Here's how the part is built. I have some questions about the finished solid (model axes, mm). Round coordinates to 2 decimals unless told otherwise and drop trailing zeros. One line per item, written item: value. Start each with the question number.
```python
from build123d import *

# Parameters (mm, degrees)
SKETCH1_R           = 25
SKETCH1_R_2         = 3.75
SKETCH1_W           = 3.2
SKETCH1_H           = 1.7
BOSS_EXTRUDE1_DEPTH = 1
FILLET1_R           = 2
FILLET2_R           = 1


with BuildPart() as part:
    # Sketch1 → Boss-Extrude1 (new body)
    with BuildSketch(Plane(origin=(0, 0, 0), x_dir=(1, 0, 0), z_dir=(0, 1, 0))):
        with Locations(Location((0, 0, 0), (0, 0, 270))):
            Circle(SKETCH1_R)
        with Locations(Location((0, 0, 0), (0, 0, 270))):
            Circle(SKETCH1_R_2, mode=Mode.SUBTRACT)
        with BuildLine():
            Line((-5, -11.456439237), (-5, -16.770509831))
            ThreePointArc((-5, -16.770509831), (0, 17.5), (5, -16.770509831))
            Line((5, -16.770509831), (5, -11.456439237))
            ThreePointArc((5, -11.456439237), (0, 12.5), (-5, -11.456439237))
        make_face(mode=Mode.SUBTRACT)
        with Locations((0, -7.85)):
            Rectangle(SKETCH1_W, SKETCH1_H, mode=Mode.SUBTRACT)
    extrude(amount=BOSS_EXTRUDE1_DEPTH)

    # Fillet1
    fillet1_edges = [part.edges().sort_by_distance(p)[0] for p in [
        (-5, 0.5, 11.456439237),
        (5, 0.5, 11.456439237),
        (5, 0.5, 16.770509831),
        (-5, 0.5, 16.770509831),
    ]]
    fillet(fillet1_edges, radius=FILLET1_R)

    # Fillet2
    fillet2_edges = [part.edges().sort_by_distance(p)[0] for p in [
        (5.952730124, 0, 15.533202189),
        (5, 0, 13.263870893),
        (5.277932277, 0, 11.681329844),
        (0, 0, -12.5),
        (-5.277932277, 0, 11.681329844),
        (-5, 0, 13.263870893),
        (-5.952730124, 0, 15.533202189),
        (0, 0, -17.5),
        (0, 0, -25),
    ]]
    fillet(fillet2_edges, radius=FILLET2_R - 0.0001)  # a hair under: the kernel refuses the full size


solid = part.part
```
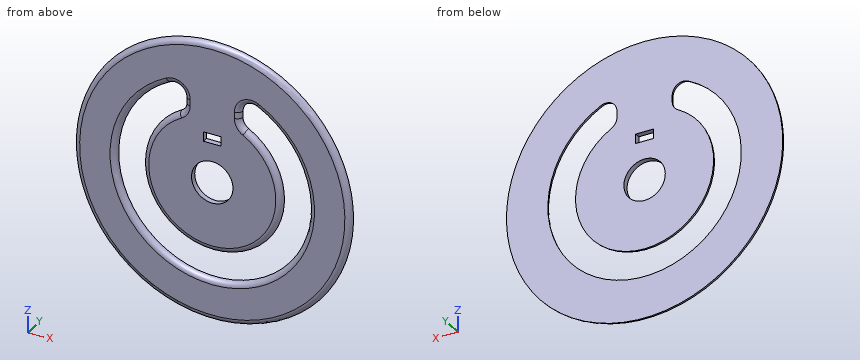
Q1. Will these pins go through, and if not, where does the flat tip stop? P1, Ø12, axis at x = 14, z = -6, coming from the +Y side; P2, Ø0.5, axis at y = 0.5, z = 8, coming from the -X side.
Q2. I want a section at A-A on x = 0. State how many separate pieces and enclosed holes the cut face has, plus the area to 3 significant figures.
Q3. If I drill on line 1 along X through (y, z) = (0.85, 0); line 2 along Z through (x, y) = (1, 0.55); line 3 along X through (y, z) = (0.45, 0), over which ranges is the centre line in solid material (lowest first)?
Answers below:
1. P1: stops at y = 1
1. P2: stops at x = -23.69
2. separate pieces: 4
2. enclosed holes: 0
2. area: 34.9 mm^2
3. line 1: x = -24.99 to -17.51, -12.49 to -3.75, 3.75 to 12.49, 17.51 to 24.99
3. line 2: z = -24.87 to -17.58, -12.35 to -3.61, 3.61 to 7, 8.7 to 24.87
3. line 3: x = -24.84 to -17.66, -12.34 to -3.75, 3.75 to 12.34, 17.66 to 24.84
